The model under review builds one solid part; all positions refer to its coordinate system, in mm. A direction names the side the tool comes from. Round coordinates to 2 decimals unless told otherwise and drop trailing zeros. Write each loop counter-clockwise with the first axis right and the second up, starting at its lowest first coordinate (ties: lowest second). Pieces come first, ordered by that corner, then holes. Notation, with made-up numbers: (67, 28) -> (112, 28) arc R14 ccw to (112, 55) -> close; hole circle Ø5 at (-12, -33). An arc over 180 degrees is marked (long way). Use CSV: the item, a comma, the result in double quotes. Start each with the question number.
1) For pin 1 Ø5 at (x, y) = (-13, 7) entering from +Z; pin 2 Ø4 at (x, y) = (17.5, 5) entering from +Z; pin 3 Ø2.5 at (x, y) = (-17.5, 4.5) entering from +Z, all flat-tipped, find the tip position at first contact; note any pin that passes through.
2) Take a section at A-A, the plane z = -7.5. Give the boundary of the cut face in (x, y), then the cut area to 3 significant figures.
3) Take a section at B-B, the plane x = 0. Give the boundary of the cut face in (y, z), then the cut area to 3 significant figures.
4) Take a section at D-D, the plane y = 20.75. State how many separate pieces and enclosed holes the cut face has, then the cut area to 3 significant figures.
5) Take a section at C-C, the plane y = 5. Give the boundary of the cut face in (x, z), then the cut area to 3 significant figures.
6) Machinability: for faces 5 (the face through (23, 13.38, -7.83)), 6 (the face through (-18, 5, -1.1)), 7 (the face through (16, 11, 4.9)), 8 (the face through (-24, 17, -6.052)), which of the approach directions +Z, -Z, +X, -X, +Y, -Y give a long, thin tool a straight path to every point of the face, cutting with its end or side? Answer none if there is none.
7) Wall thickness on probe 1 along Y at (x, z) = (27.5, -2.2); probe 2 along X at (y, z) = (5, 3.55); probe 3 along Y at (x, z) = (29, -3.5): over which ranges is each line inside the solid? List them lowest first. Write a range as [from, to].
8) Mouldability with a two-part tool opening along X and no side actions: class faces 1 (the face through (0, 11, -5.1)), 2 (the face through (35, 9, 0)), 3 (the face through (-8, 23, 9.9)), 4 (the face through (-32.861, 22.745, 0.089)) as released by +X, released by -X, zero draft, split by the parting line, or undercut.
from build123d import *

# Parameters (mm, degrees)
BOSS_EXTRUDE1_DEPTH                             = 25
SKETCH2_R                                       = 2.45
CUT_EXTRUDE1_DEPTH                              = 25
FILLET1_R                                       = 7.5
SKETCH3_W                                       = 55
SKETCH3_H                                       = 19.9
BOSS_EXTRUDE2_DEPTH                             = 3
CSK_FOR_M2_FLAT_HEAD_MACHINE_SCREW1_D           = 2.4
CSK_FOR_M2_FLAT_HEAD_MACHINE_SCREW1_DEPTH       = 10
CSK_FOR_M2_FLAT_HEAD_MACHINE_SCREW1_CSINK_D     = 6.4
CSK_FOR_M2_FLAT_HEAD_MACHINE_SCREW1_CSINK_ANGLE = 90
CSK_FOR_M2_FLAT_HEAD_MACHINE_SCREW1_TIP         = 0.721032743
FILLET2_R                                       = 0.5
CSK_FOR_M5_FLAT_HEAD_MACHINE_SCREW1_D           = 5.1
CSK_FOR_M5_FLAT_HEAD_MACHINE_SCREW1_DEPTH       = 6
CSK_FOR_M5_FLAT_HEAD_MACHINE_SCREW1_CSINK_D     = 5.5
CSK_FOR_M5_FLAT_HEAD_MACHINE_SCREW1_CSINK_ANGLE = 70


with BuildPart() as part:
    # Sketch1 → Boss-Extrude1 (new body)
    with BuildSketch(Plane(origin=(0, 0, 0), x_dir=(1, 0, 0), z_dir=(0, 1, 0))):
        Polygon((-35, 10), (-35, -9.9), (-23.097924618, -9.9), (-23.097924618, -5), (-23.097924618, -4.9), (-22.997924618, -4.9), (-8.190022831, -4.9), (-15.192098213, 5.1), (15.192098213, 5.1), (8.190022831, -4.9), (22.997924618, -4.9), (23.097924618, -4.9), (23.097924618, -5), (23.097924618, -9.9), (35, -9.9), (35, 10), align=None)
    extrude(amount=BOSS_EXTRUDE1_DEPTH)

    # Sketch2 → Cut-Extrude1 (cut)
    with BuildSketch(Plane(origin=(0, 0, -10), x_dir=(-1, 0, 0), z_dir=(0, 0, -1))):
        with Locations((-27.5, 17.5)):
            Circle(SKETCH2_R)
        with Locations((27.5, 17.5)):
            Circle(SKETCH2_R)
    extrude(amount=-CUT_EXTRUDE1_DEPTH, mode=Mode.SUBTRACT)

    # Fillet1
    fillet1_edges = [part.edges().sort_by_distance(p)[0] for p in [
        (35, 25, -0.05),
        (-35, 25, -0.05),
    ]]
    fillet(fillet1_edges, radius=FILLET1_R)

    # Sketch3 → Boss-Extrude2 (add)
    with BuildSketch(Plane(origin=(0, 25, 0), x_dir=(1, 0, 0), z_dir=(0, 1, 0))):
        with Locations((0, 0.05)):
            Rectangle(SKETCH3_W, SKETCH3_H)
    extrude(amount=-BOSS_EXTRUDE2_DEPTH)

    # CSK for M2 Flat Head Machine Screw1
    with Locations(Plane(origin=(0, 22, 0), x_dir=(-1, 0, 0), z_dir=(0, -1, 0))):
        with Locations((0, 0)):
            CounterSinkHole(CSK_FOR_M2_FLAT_HEAD_MACHINE_SCREW1_D / 2, CSK_FOR_M2_FLAT_HEAD_MACHINE_SCREW1_CSINK_D / 2, depth=CSK_FOR_M2_FLAT_HEAD_MACHINE_SCREW1_DEPTH, counter_sink_angle=CSK_FOR_M2_FLAT_HEAD_MACHINE_SCREW1_CSINK_ANGLE)
            with Locations((0, 0, -(CSK_FOR_M2_FLAT_HEAD_MACHINE_SCREW1_DEPTH + CSK_FOR_M2_FLAT_HEAD_MACHINE_SCREW1_TIP / 2))):  # 118° drill point
                Cone(0, CSK_FOR_M2_FLAT_HEAD_MACHINE_SCREW1_D / 2, CSK_FOR_M2_FLAT_HEAD_MACHINE_SCREW1_TIP, mode=Mode.SUBTRACT)

    # Fillet2
    fillet2_edges = [part.edges().sort_by_distance(p)[0] for p in [
        (8.190022831, 11, 4.9),
        (-8.190022831, 11, 4.9),
    ]]
    fillet(fillet2_edges, radius=FILLET2_R)

    # Sketch10 → Cut-Revolve1 (revolve, cut)
    with BuildSketch(Plane(origin=(0, 17.5, 0), x_dir=(1, 0, 0), z_dir=(0, 1, 0)), mode=Mode.PRIVATE) as cut_revolve1_sk:
        Polygon((-27.5, 6.052481049), (-27.5, 10.005610284), (-33.6, 10.005610284), (-33.6, 5.605610284), (-32.25, 5.213190854), (-32.25, 0.052481049), (-31.453797848, 0.052481049), (-31.453797848, 6.052481049), (-30.701898924, 6.052481049), (-31.453797848, 6.784043238), (-31.453797848, 9.993311616), (-29.95, 9.993311616), (-29.95, 6.052481049), (-29.95, 0.052481049), (-27.5, 0.052481049), align=None)
    revolve(cut_revolve1_sk.sketch.rotate(Axis((-27.5, 17.5, 990.182204964), (0, 0, -1)), 180), axis=Axis((-27.5, 17.5, 990.182204964), (0, 0, -1)), mode=Mode.SUBTRACT)

    # Sketch10_3 → Cut-Revolve2 (revolve, cut)
    with BuildSketch(Plane(origin=(0, 17.5, 0), x_dir=(1, 0, 0), z_dir=(0, 1, 0))):
        Polygon((31.453797848, 9.993311616), (31.453797848, 6.784043238), (30.701898924, 6.052481049), (31.453797848, 6.052481049), (31.453797848, 0.052481049), (32.25, 0.052481049), (32.25, 5.213190854), (33.6, 5.605610284), (33.6, 10.005610284), (27.5, 10.005610284), (27.5, 6.052481049), (27.5, 0.052481049), (29.95, 0.052481049), (29.95, 6.052481049), (29.95, 9.993311616), align=None)
    revolve(axis=Axis((27.5, 17.5, 990.028974512), (0, 0, -1)), mode=Mode.SUBTRACT)

    # CSK for M5 Flat Head Machine Screw1
    with Locations(Plane.XY.offset(4.9)):
        with Locations((-18.097924618, 5), (18.097924618, 5)):
            CounterSinkHole(CSK_FOR_M5_FLAT_HEAD_MACHINE_SCREW1_D / 2, CSK_FOR_M5_FLAT_HEAD_MACHINE_SCREW1_CSINK_D / 2, depth=CSK_FOR_M5_FLAT_HEAD_MACHINE_SCREW1_DEPTH, counter_sink_angle=CSK_FOR_M5_FLAT_HEAD_MACHINE_SCREW1_CSINK_ANGLE)


solid = part.part
Values found:
1,pin 1,"z = 4.9"
1,pin 2,"z = 4.68"
1,pin 3,"z = -1.1"
2,outline,"(-35, 0) -> (35, 0) -> (35, 17.5) arc R7.5 ccw to (27.5, 25) -> (-27.5, 25) arc R7.5 ccw to (-35, 17.5) -> close; circle Ø7.91 at (-27.5, 17.5); circle Ø7.91 at (27.5, 17.5); hole circle Ø12.2 at (-27.5, 17.5); hole circle Ø4.9 at (-27.5, 17.5); hole circle Ø12.2 at (27.5, 17.5); hole circle Ø4.9 at (27.5, 17.5)"
2,area,"1,550 mm²"
3,outline,"(0, -10) -> (25, -10) -> (25, -1.2) -> (24, -1.2) -> (22, -3.2) -> (22, -5.1) -> (0, -5.1) -> close; (22, 3.2) -> (24, 1.2) -> (25, 1.2) -> (25, 9.9) -> (22, 9.9) -> close"
3,area,"156 mm²"
4,separate pieces,"3"
4,enclosed holes,"0"
4,area,"816 mm²"
5,outline,"(-35, -10) -> (35, -10) -> (35, 9.9) -> (23.1, 9.9) -> (23.1, 4.9) -> (20.85, 4.9) -> (20.65, 4.61) -> (20.65, -1.1) -> (15.55, -1.1) -> (15.55, 4.61) -> (15.35, 4.9) -> (9.15, 4.9) arc R0.5 ccw to (8.74, 4.11) -> (15.19, -5.1) -> (-15.19, -5.1) -> (-8.74, 4.11) arc R0.5 ccw to (-9.15, 4.9) -> (-15.35, 4.9) -> (-15.55, 4.61) -> (-15.55, -1.1) -> (-20.65, -1.1) -> (-20.65, 4.61) -> (-20.85, 4.9) -> (-23.1, 4.9) -> (-23.1, 9.9) -> (-35, 9.9) -> close"
5,area,"866 mm²"
6,face 5,"-Z"
6,face 6,"+Z"
6,face 7,"+Z, -Y"
6,face 8,"none"
7,probe 1,"[0, 12.75], [13.55, 15.05], [19.95, 21.45], [22.25, 25]"
7,probe 2,"[-35, -20.65], [-15.55, -9.14], [9.14, 15.55], [20.65, 35]"
7,probe 3,"[0, 12.99], [13.84, 15.56], [19.44, 21.16], [22.01, 24.85]"
8,face 1,"undercut"
8,face 2,"released by +X"
8,face 3,"zero draft"
8,face 4,"released by -X"
